Job drawing, mm, ordinate dimensions from the low corner. One solid piece. Give positions to 0.01 mm unless a question says otherwise; leave off trailing zeros. Loops run counter-clockwise (first coordinate to the right, second up) from the corner with the lowest first, then second, coordinate; pieces in that order, holes last. Notation, with made-up numbers: (0, 46.5) -> (36, 46.5) arc R16 ccw to (36, 67.5) -> close; hole circle Ø1 at (-36, 6). An arc over 180 degrees is marked (long way). Use one line per item in the form item = value.
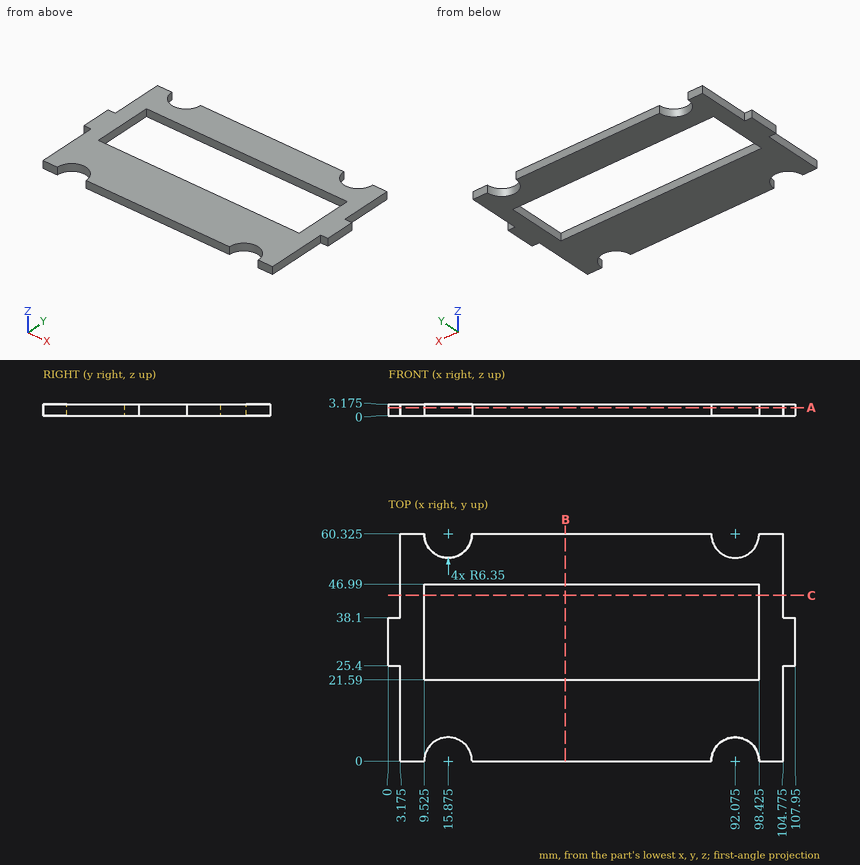
1. Cut at C-C, the plane y = 44. Write the cut outline in (x, z) (3 decimals), then the cut area to 3 significant figures.
Result sheet:
outline = (3.175, 0) -> (9.525, 0) -> (9.525, 3.175) -> (3.175, 3.175) -> close; (98.425, 0) -> (104.775, 0) -> (104.775, 3.175) -> (98.425, 3.175) -> close
area = 40.3 mm^2
2. Cut at A-A, the plane z = 2.2. Write the cut outline in (x, y) (3 decimals).
Result sheet:
outline = (0, 25.4) -> (3.175, 25.4) -> (3.175, 0) -> (9.525, 0) arc R6.35 cw to (22.225, 0) -> (85.725, 0) arc R6.35 cw to (98.425, 0) -> (104.775, 0) -> (104.775, 25.4) -> (107.95, 25.4) -> (107.95, 38.1) -> (104.775, 38.1) -> (104.775, 60.325) -> (98.425, 60.325) arc R6.35 cw to (85.725, 60.325) -> (22.225, 60.325) arc R6.35 cw to (9.525, 60.325) -> (3.175, 60.325) -> (3.175, 38.1) -> (0, 38.1) -> close; hole (9.525, 21.59) -> (98.425, 21.59) -> (98.425, 46.99) -> (9.525, 46.99) -> close
3. Drill centre lines: line 1 (Y direction, x = 33, z = 1.1) (3 decimals); line 2 (X direction, y = 27.5, z = 2.9) (3 decimals); line 3 (X direction, y = 56, z = 2.2) (3 decimals). Where is each one in solid material? Low to high.
Result sheet:
line_1 = 0 to 21.59, 46.99 to 60.325
line_2 = 0 to 9.525, 98.425 to 107.95
line_3 = 3.175 to 11.226, 20.524 to 87.426, 96.724 to 104.775
4. Drop flat-ended pins along their axis: P1, Ø1.6, axis at y = 54.5, z = 1, coming from the -X side (3 decimals); P2, Ø1, axis at y = 44, z = 2, coming from the +X side (3 decimals); P3, Ø1.6, axis at x = 1, z = 2.5, coming from the +Y side. Give the stop position or say it passes through.
Result sheet:
P1 = 3.175
P2 = 104.775
P3 = 38.1
5. Cut at B-B, the plane x = 47. Write the cut outline in (y, z) (3 decimals), then the cut area to 3 significant figures.
Result sheet:
outline = (0, 0) -> (21.59, 0) -> (21.59, 3.175) -> (0, 3.175) -> close; (46.99, 0) -> (60.325, 0) -> (60.325, 3.175) -> (46.99, 3.175) -> close
area = 111 mm^2
